from build123d import *

# Parameters (mm, degrees)
BOX_W           = 60
BOX_H           = 70
BOX_DEPTH       = 60
PRISM001_DEPTH  = 60
PRISM_DEPTH     = 60
SKETCH_R        = 8
POCKET_DEPTH    = 2
SKETCH001_R     = 8
POCKET001_DEPTH = 2
SKETCH002_R     = 8
POCKET002_DEPTH = 2
SKETCH003_R     = 8
POCKET003_DEPTH = 2
SKETCH004_W     = 16.007478
SKETCH004_H     = 3
PAD_DEPTH       = 10
SKETCH005_W     = 11.852036
SKETCH005_H     = 3
PAD001_DEPTH    = 10
SKETCH006_R     = 3.1
POCKET004_DEPTH = 5
SKETCH007_R     = 3.1
POCKET005_DEPTH = 5


with BuildPart() as cubo:
    # Box → Box (new body)
    with BuildSketch(Plane(origin=(0, -35, 0), x_dir=(1, 0, 0), z_dir=(0, 0, 1))):
        with Locations((30, 35)):
            Rectangle(BOX_W, BOX_H)
    extrude(amount=BOX_DEPTH)


with BuildPart() as prisma001:
    # Prism001 → Prism001 (new body)
    with BuildSketch(Plane.XY):
        Polygon((31, 0), (21.9203102168, 21.9203102168), (0, 31), (-21.9203102168, 21.9203102168), (-31, 0), (-21.9203102168, -21.9203102168), (0, -31), (21.9203102168, -21.9203102168), align=None)
    extrude(amount=PRISM001_DEPTH)


with BuildPart() as pocket005:
    # Prism → Prism (new body)
    with BuildSketch(Plane.XY):
        Polygon((32.5, 0), (22.9809703886, 22.9809703886), (0, 32.5), (-22.9809703886, 22.9809703886), (-32.5, 0), (-22.9809703886, -22.9809703886), (0, -32.5), (22.9809703886, -22.9809703886), align=None)
    extrude(amount=PRISM_DEPTH)

    # Cut: cut Prisma001
    add(prisma001.part, mode=Mode.SUBTRACT)

    # Cut001: cut Cubo
    add(cubo.part, mode=Mode.SUBTRACT)

    # Sketch → Pocket (cut)
    with BuildSketch(Plane(origin=(-11.4904851943, -27.7404851943, 0), x_dir=(0.9238795325, -0.3826834324, 0), z_dir=(-0.3826834324, -0.9238795325, 0))):
        with Locations((0, 48)):
            Circle(SKETCH_R)
        with Locations((0, 22)):
            Circle(SKETCH_R)
    extrude(amount=-POCKET_DEPTH, mode=Mode.SUBTRACT)

    # Sketch001 → Pocket001 (cut)
    with BuildSketch(Plane(origin=(-27.7404851943, -11.4904851943, 0), x_dir=(0.3826834324, -0.9238795325, 0), z_dir=(-0.9238795325, -0.3826834324, 0))):
        with Locations((0, 48)):
            Circle(SKETCH001_R)
        with Locations((0, 22)):
            Circle(SKETCH001_R)
    extrude(amount=-POCKET001_DEPTH, mode=Mode.SUBTRACT)

    # Sketch002 → Pocket002 (cut)
    with BuildSketch(Plane(origin=(-27.7404851943, 11.4904851943, 0), x_dir=(-0.3826834324, -0.9238795325, 0), z_dir=(-0.9238795325, 0.3826834324, 0))):
        with Locations((0, 48)):
            Circle(SKETCH002_R)
        with Locations((0, 22)):
            Circle(SKETCH002_R)
    extrude(amount=-POCKET002_DEPTH, mode=Mode.SUBTRACT)

    # Sketch003 → Pocket003 (cut)
    with BuildSketch(Plane(origin=(-11.4904851943, 27.7404851943, 0), x_dir=(-0.9238795325, -0.3826834324, 0), z_dir=(-0.3826834324, 0.9238795325, 0))):
        with Locations((6e-06, 48)):
            Circle(SKETCH003_R)
        with Locations((0, 22)):
            Circle(SKETCH003_R)
    extrude(amount=-POCKET003_DEPTH, mode=Mode.SUBTRACT)

    # Sketch004 → Pad (new body)
    with BuildSketch(Plane(origin=(-27.7404851943, 11.4904851943, 0), x_dir=(-0.3826834324, -0.9238795325, 0), z_dir=(-0.9238795325, 0.3826834324, 0))):
        with Locations((4.178784, 1.5)):
            Rectangle(SKETCH004_W, SKETCH004_H)
    extrude(amount=PAD_DEPTH)

    # Sketch005 → Pad001 (new body)
    with BuildSketch(Plane(origin=(-27.7404851943, -11.4904851943, 0), x_dir=(0.3826834324, -0.9238795325, 0), z_dir=(-0.9238795325, -0.3826834324, 0))):
        with Locations((-6.240987, 1.5)):
            Rectangle(SKETCH005_W, SKETCH005_H)
    extrude(amount=PAD001_DEPTH)

    # Sketch006 → Pocket004 (cut)
    with BuildSketch(Plane.XY.offset(3)):
        with Locations((-34.283413, 8.452291)):
            Circle(SKETCH006_R)
    extrude(amount=-POCKET004_DEPTH, mode=Mode.SUBTRACT)

    # Sketch007 → Pocket005 (cut)
    with BuildSketch(Plane.XY.offset(3)):
        with Locations((-35.295174, -6.471159)):
            Circle(SKETCH007_R)
    extrude(amount=-POCKET005_DEPTH, mode=Mode.SUBTRACT)


solid = pocket005.part
Geometry: final body of the model. Coordinates: model frame, mm. A direction names the side the tool comes from. Round coordinates to 2 decimals unless told otherwise and drop trailing zeros. Write each loop counter-clockwise with the first axis right and the second up, starting at its lowest first coordinate (ties: lowest second). Pieces come first, ordered by that corner, then holes. Notation, with made-up numbers: M 84,59.5 L 118,59.5 A9 cw 118,65.5 Z; hole C 7.5,86 d6. An arc over 180 degrees is marked long. Write item = value, one per line.
Item 1: Material intervals for line 1 along Y through (x, z) = (-9, 9.5); line 2 along Z through (x, y) = (-31.5, -7.5); line 3 along Y through (x, z) = (-22, 29), sorted ascending. Write a range as [from, to].
Findings:
line_1 = [-28.77, -27.27], [27.27, 28.77]
line_2 = [0, 3]
line_3 = [-23.39, -21.73], [21.73, 23.39]
Item 2: Section query D-D on y = 7.5. State how many separate pieces and enclosed holes the cut face has, then the cut area to 3 significant figures.
Findings:
separate_pieces = 4
enclosed_holes = 0
area = 63.3 mm^2
Item 3: Section query C-C on z = 19. Return loops of the section in (x, y).
Findings:
outline = M -32.5,0 L -30.58,-4.64 L -29.3,-4.11 L -31,0 L -29.3,4.11 L -30.58,4.64 Z; M -24.9,-18.34 L -22.98,-22.98 L -18.34,-24.9 L -17.81,-23.62 L -21.92,-21.92 L -23.62,-17.81 Z; M -24.9,18.34 L -23.62,17.81 L -21.92,21.92 L -17.81,23.62 L -18.34,24.9 L -22.98,22.98 Z; M -4.64,-30.58 L 0,-32.5 L 0,-31 L -4.11,-29.3 Z; M -4.64,30.58 L -4.11,29.3 L 0,31 L 0,32.5 Z
Item 4: Section query A-A on z = 5.5. Return loops of the section in (x, y), then the cut area to 3 significant figures.
Findings:
outline = M -32.5,0 L -22.98,-22.98 L 0,-32.5 L 0,-31 L -21.92,-21.92 L -31,0 L -21.92,21.92 L 0,31 L 0,32.5 L -22.98,22.98 Z
area = 135 mm^2
Item 5: Pin query (flat end, axial travel): P1, Ø5.5, axis at x = -34.28, y = 8.45, coming from the -Z side; P2, Ø4, axis at x = -34, y = -8.5, coming from the +Z side; P3, Ø5, axis at x = -8.5, z = 34.5, coming from the -Y side; P4, Ø6, axis at y = -4, z = 34, coming from the -X side. Return the tip coordinate at first contact, or that it passes through.
Findings:
P1 = through
P2 = 3
P3 = -30.01
P4 = -32.09
Item 6: Section query B-B on x = -2.5. Return loops of the section in (y, z), then the cut area to 3 significant figures.
Findings:
outline = M -31.46,0 L -29.96,0 L -29.96,60 L -31.46,60 Z; M 29.96,0 L 31.46,0 L 31.46,60 L 29.96,60 Z
area = 180 mm^2
Item 7: Pull-direction query (Z, two-part tool) for faces 4 (the face through (-36.951, -2.136, 1.479)), 5 (the face through (-12.191, -26.711, 29.932)), 6 (the face through (-32, 11, 3)); classes: pulls with the +Z half, pulls with the -Z half, needs draft (parallel to the pull), parting line crosses it, or undercut.
Findings:
face_4 = needs draft
face_5 = undercut
face_6 = pulls with the +Z half
Item 8: Access query for faces 1 (the face through (-30.8, 16.9, 1.5)), 2 (the face through (-34, -10, 3)), 3 (the face through (-5.94, 28.54, 29.58)). Directions: +Z, -Z, +X, -X, +Y, -Y. A direction counts if a zero-diameter tool reaches every point of the face in a straight line with its end or side. Return the directions, or none.
Findings:
face_1 = +Z, -Z, +Y
face_2 = +Z, -X, -Y
face_3 = +Z, -Z, +X
